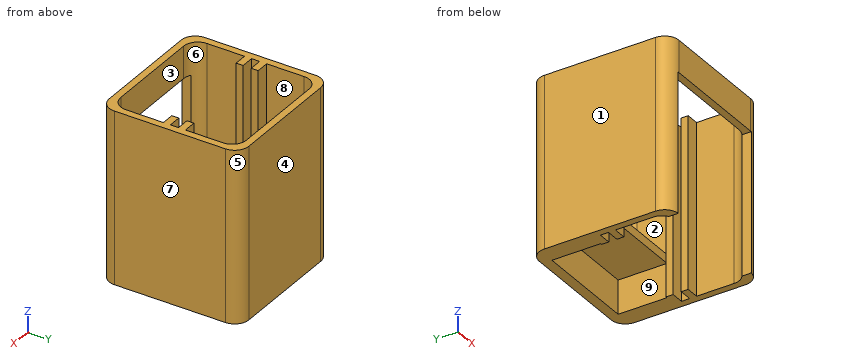
```python
from build123d import *

# Parameters (mm, degrees)
SKETCH1_W           = 100
SKETCH1_H           = 100
BOSS_EXTRUDE1_DEPTH = 250
SKETCH2_W           = 90
SKETCH2_H           = 90
CUT_EXTRUDE1_DEPTH  = 288.228132327
FILLET1_R           = 10.16
SKETCH3_W           = 9.3412
SKETCH3_H           = 5
BOSS_EXTRUDE2_DEPTH = 250
SKETCH4_W           = 100
SKETCH4_H           = 125
CUT_EXTRUDE2_DEPTH  = 288.228132327
SKETCH6_W           = 81
SKETCH6_H           = 100
CUT_EXTRUDE4_DEPTH  = 5
FILLET3_R           = 10.16
BOSS_EXTRUDE3_DEPTH = 30.48
SKETCH9_W           = 73.406
SKETCH9_H           = 6.25
BOSS_EXTRUDE5_DEPTH = 35.052
CUT_EXTRUDE5_DEPTH  = 2


with BuildPart() as part:
    # Sketch1 → Boss-Extrude1 (new body)
    with BuildSketch(Plane.XY):
        with Locations((50, 50)):
            Rectangle(SKETCH1_W, SKETCH1_H)
    extrude(amount=BOSS_EXTRUDE1_DEPTH)

    # Sketch2 → Cut-Extrude1 (cut, through all)
    with BuildSketch(Plane(origin=(0, 0, 0), x_dir=(-1, 0, 0), z_dir=(0, 0, -1))):
        with Locations((-50, 50)):
            Rectangle(SKETCH2_W, SKETCH2_H)
    extrude(amount=-CUT_EXTRUDE1_DEPTH, mode=Mode.SUBTRACT)

    # Fillet1
    fillet1_edges = [part.edges().sort_by_distance(p)[0] for p in [
        (0, 100, 125),
        (0, 0, 125),
        (100, 0, 125),
        (100, 100, 125),
    ]]
    fillet(fillet1_edges, radius=FILLET1_R)

    # Sketch3 → Boss-Extrude2 (add, through all)
    with BuildSketch(Plane(origin=(0, 0, 0), x_dir=(-1, 0, 0), z_dir=(0, 0, -1))):
        with Locations((-90.3294, 55.4)):
            Rectangle(SKETCH3_W, SKETCH3_H)
        with Locations((-90.3294, 44.6)):
            Rectangle(SKETCH3_W, SKETCH3_H)
        with Locations((-9.6706, 44.6)):
            Rectangle(SKETCH3_W, SKETCH3_H)
        with Locations((-9.6706, 55.4)):
            Rectangle(SKETCH3_W, SKETCH3_H)
    extrude(amount=-BOSS_EXTRUDE2_DEPTH)

    # Sketch4 → Cut-Extrude2 (cut, through all)
    with BuildSketch(Plane(origin=(0, 100, 0), x_dir=(1, 0, 0), z_dir=(0, 1, 0))):
        with Locations((50, -62.5)):
            Rectangle(SKETCH4_W, SKETCH4_H)
    extrude(amount=-CUT_EXTRUDE2_DEPTH, mode=Mode.SUBTRACT)

    # Sketch6 → Cut-Extrude4 (cut)
    with BuildSketch(Plane.XZ):
        with Locations((50, 175)):
            Rectangle(SKETCH6_W, SKETCH6_H)
    extrude(amount=-CUT_EXTRUDE4_DEPTH, mode=Mode.SUBTRACT)

    # Fillet3
    fillet3_edges = [part.edges().sort_by_distance(p)[0] for p in [
        (5, 95, 187.5),
        (5, 5, 187.5),
        (95, 95, 187.5),
        (95, 5, 187.5),
    ]]
    fillet(fillet3_edges, radius=FILLET3_R)

    # Sketch7 → Boss-Extrude3 (add)
    with BuildSketch(Plane(origin=(0, 0, 125), x_dir=(-1, 0, 0), z_dir=(0, 0, -1))):
        Polygon((-95, 96), (-5, 96), (-5, 57.9), (-13.297, 57.9), (-13.297, 92.952), (-86.703, 92.952), (-86.703, 57.9), (-95, 57.9), align=None)
    extrude(amount=-BOSS_EXTRUDE3_DEPTH)

    # Sketch9 → Boss-Extrude5 (add)
    with BuildSketch(Plane.XZ.offset(-92.952)):
        with Locations((50, 152.355)):
            Rectangle(SKETCH9_W, SKETCH9_H)
    extrude(amount=BOSS_EXTRUDE5_DEPTH)

    # Sketch10 → Cut-Extrude5 (cut)
    with BuildSketch(Plane.XY.offset(250)):
        with BuildLine():
            Line((89.84, 100), (10.16, 100))
            ThreePointArc((10.16, 100), (2.975795103, 97.024204897), (0, 89.84))
            Line((0, 89.84), (0, 10.16))
            ThreePointArc((0, 10.16), (2.975795103, 2.975795103), (10.16, 0))
            Line((10.16, 0), (89.84, 0))
            ThreePointArc((89.84, 0), (97.024204897, 2.975795103), (100, 10.16))
            Line((100, 10.16), (100, 89.84))
            ThreePointArc((100, 89.84), (97.024204897, 97.024204897), (89.84, 100))
        make_face()
    extrude(amount=-CUT_EXTRUDE5_DEPTH, mode=Mode.SUBTRACT)


solid = part.part
```
Geometry check sheet. Reference: the model listing, model coordinates, mm. Face numbers are marked on the shaded views. A direction names the side the tool comes from. Coordinates: 2 decimals unless noted, no trailing zeros. Order: outer loops, then holes, each group sorted by start corner. A loop starts at its lowest first (then second) coordinate and runs counter-clockwise, first axis right, second up. Notation, with made-up numbers: (-32.5, 5.5) - (24.5, 5.5) arc R28 cw to (24.5, 27.5) - close; hole circle Ø3 at (-9, 69). An arc over 180 degrees is marked (long way). Answer as a JSON object with one key per item and string values. Group by question number.
Item 1: Sectioned sample at D-D, the plane y = 70.5. Record the cut outline in (x, z).
Item 2: Draft check along X on the marked faces 1, 2, 3 and 4. Enter one of: +X half, -X half, draft (parallel to the pull), parting line (faces both ways), or undercut.
Item 3: Depth check by flat-ended pin: pin 1 Ø7.5 at (x, z) = (10, 194) entering from -Y; pin 2 Ø12 at (x, z) = (32.5, 141.5) entering from -Y; pin 3 Ø1 at (x, y) = (80, 59) entering from -Z. Enter the tip coordinate at first touch or a pass-through.
Item 4: Sectioned sample at B-B, the plane x = 66.5. Record the cut outline in (y, z), and give its area (3 significant figures).
Item 5: Scan lines: probe 1 along Y at (x, z) = (86, 232); probe 2 along Y at (x, z) = (73.5, 229). Record each from-to range of solid material in increasing order.
Item 6: Tool access check on the marked faces 5, 6, 7, 8 and 9. Record the directions out of +Z, -Z, +X, -X, +Y, -Y that give a thin tool (end or side, any length) a straight path to the whole face; none if there is none.
Item 7: Sectioned sample at A-A, the plane y = 56. Record the cut outline in (x, z), and give its area (3 significant figures).
Resolved:
{
 "1": {"outline": "(0, 125) - (13.3, 125) - (13.3, 149.23) - (86.7, 149.23) - (86.7, 125) - (100, 125) - (100, 248) - (95, 248) - (95, 155.48) - (5, 155.48) - (5, 248) - (0, 248) - close"},
 "2": {"face 1": "-X half", "face 2": "undercut", "face 3": "undercut", "face 4": "draft"},
 "3": {"pin 1": "y = 0.02", "pin 2": "y = 92.95", "pin 3": "z = 149.23"},
 "4": {"outline": "(0, 225) - (5, 225) - (5, 248) - (0, 248) - close; (57.9, 149.23) - (92.95, 149.23) - (92.95, 125) - (100, 125) - (100, 248) - (95, 248) - (95, 155.48) - (57.9, 155.48) - close", "area": "1,010 mm^2"},
 "5": {"probe 1": "0 to 5.07, 42.1 to 47.1, 52.9 to 57.9, 94.93 to 100", "probe 2": "0 to 5, 95 to 100"},
 "6": {"face 5": "+Z, -Z, +X, +Y", "face 6": "+Z, -Z", "face 7": "+Z, -Z, +X, +Y, -Y", "face 8": "+Z", "face 9": "-Z"},
 "7": {"outline": "(0, 125) - (14.34, 125) - (14.34, 248) - (0, 248) - close; (85.66, 125) - (100, 125) - (100, 248) - (85.66, 248) - close", "area": "3,530 mm^2"}
}
